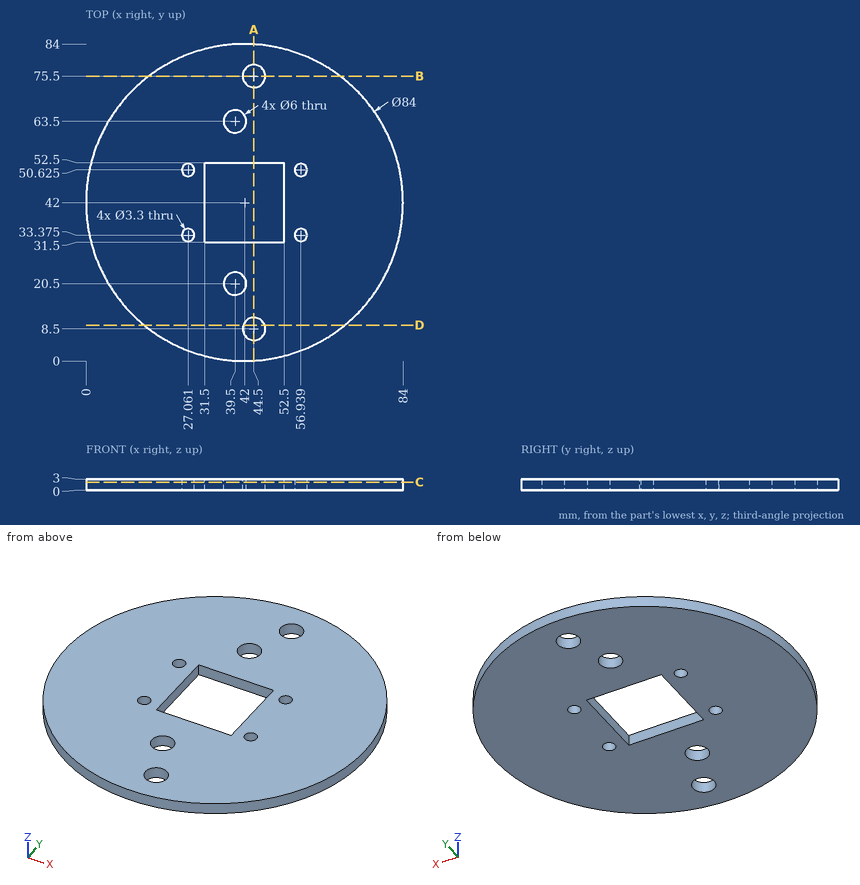
Print and shaded views of the part. All mm, measured from the part's lowest x, y and z. Coordinates: 2 decimals unless noted, no trailing zeros. Write each loop counter-clockwise with the first axis right and the second up, starting at its lowest first coordinate (ties: lowest second). Pieces come first, ordered by that corner, then holes. Notation, with made-up numbers: (11.25, 33.25) - (49.25, 33.25) arc R32 cw to (49.25, 68.25) - close; hole circle Ø1 at (-21.5, 88.5). An arc over 180 degrees is marked (long way). One line per question, with ' | ' between items. Start each with the question number.
Q1. Cut at B-B, the plane y = 75.5. List the corners of the cut face in (x, z).
Q2. Cut at A-A, the plane x = 44.5. List the corners of the cut face in (y, z).
Q3. Cut at C-C, the plane z = 2.15. Give the number of separate pieces and of enclosed holes in the cut face, then the cut area to 3 significant figures.
Q4. Cut at D-D, the plane y = 9.5. List the corners of the cut face in (x, z), then the cut area to 3 significant figures.
Q5. Pin check, flat tip, straight feed: pin 1 (1.5 mm diameter, centred on x = 43, z = 1.5, fed in from +Y). Stop position of the tip, or through.
Q6. Drill centre lines: line 1 (Y direction, x = 39.5, z = 0.7); line 2 (X direction, y = 49.5, z = 2.05) (3 decimals); line 3 (Y direction, x = 27, z = 0.15). Where is each one in solid material? Low to high. Write a range as [from, to].
Answer below:
1) outline: (16.67, 0) - (41.5, 0) - (41.5, 3) - (16.67, 3) - close; (47.5, 0) - (67.33, 0) - (67.33, 3) - (47.5, 3) - close
2) outline: (0.07, 0) - (5.5, 0) - (5.5, 3) - (0.07, 3) - close; (11.5, 0) - (31.5, 0) - (31.5, 3) - (11.5, 3) - close; (52.5, 0) - (72.5, 0) - (72.5, 3) - (52.5, 3) - close; (78.5, 0) - (83.93, 0) - (83.93, 3) - (78.5, 3) - close
3) separate pieces: 1 | enclosed holes: 9 | area: 4,950 mm^2
4) outline: (15.4, 0) - (41.67, 0) - (41.67, 3) - (15.4, 3) - close; (47.33, 0) - (68.6, 0) - (68.6, 3) - (47.33, 3) - close | area: 143 mm^2
5) pin 1: y = 84
6) line 1: [0.07, 17.5], [23.5, 31.5], [52.5, 60.5], [66.5, 83.93] | line 2: [0.675, 25.854], [28.268, 31.5], [52.5, 55.732], [58.146, 83.325] | line 3: [2.77, 31.73], [35.02, 48.98], [52.27, 81.23]
